Geometry check sheet. Reference: the model listing, model coordinates, mm. Face numbers are marked on the shaded views. A direction names the side the tool comes from. Give positions to 0.01 mm unless a question says otherwise; leave off trailing zeros. Write each loop counter-clockwise with the first axis right and the second up, starting at its lowest first coordinate (ties: lowest second). Pieces come first, ordered by that corner, then holes. Notation, with made-up numbers: M -28,9 L 10,9 A20 cw 10,35 Z; hole C 71.5,53 d8. An arc over 180 degrees is marked long. Write each question's results on one line, items separated by ' | '.
```python
from build123d import *

# Parameters (mm, degrees)
EXTRUDE1_DEPTH                   = 15.875
EXTRUDE2_DEPTH                   = 50
F_3_8_0_375_DIAMETER_HOLE1_D     = 9.525
F_3_8_0_375_DIAMETER_HOLE1_DEPTH = 32.4000114
F_3_8_0_375_DIAMETER_HOLE1_TIP   = 1.733408241
SKETCH6_R                        = 4.5
EXTRUDE3_DEPTH                   = 165.426993678


with BuildPart() as part:
    # Sketch1 → Extrude1 (new body)
    with BuildSketch(Plane(origin=(0, 0, 0), x_dir=(0, 0, -1), z_dir=(1, 0, 0))):
        with BuildLine():
            Line((0, 0), (-155.575, 0))
            Line((-155.575, 0), (-155.575, 14.6939))
            Line((-155.575, 14.6939), (-76.581, 14.6939))
            ThreePointArc((-76.581, 14.6939), (-69.845807909, 17.483707909), (-67.056, 24.2189))
            Line((-67.056, 24.2189), (-67.056, 25.4254))
            ThreePointArc((-67.056, 25.4254), (-69.845807909, 32.160592091), (-76.581, 34.9504))
            Line((-76.581, 34.9504), (-89.706369343, 34.9504))
            Line((-89.706369343, 34.9504), (-92.456, 36.5379))
            Line((-92.456, 36.5379), (-92.456, 49.2125))
            Line((-92.456, 49.2125), (-89.706369343, 50.8))
            Line((-89.706369343, 50.8), (0, 50.8))
            Line((0, 50.8), (0, 0))
        make_face()
    extrude(amount=EXTRUDE1_DEPTH)

    # Sketch2 → Extrude2 (cut)
    with BuildSketch(Plane.XY.offset(155.575)):
        Polygon((0, 10.9855), (4.462954262, 10.9855), (6.604, 14.6939), (9.271, 14.6939), (11.412045738, 10.9855), (15.875, 10.9855), (15.875, 23.6855), (0, 23.6855), align=None)
    extrude(amount=-EXTRUDE2_DEPTH, mode=Mode.SUBTRACT)

    # Sketch3 → Cut-Revolve1 (revolve, cut)
    with BuildSketch(Plane.XY.offset(105.575)):
        Polygon((0, 10.9855), (4.462954262, 10.9855), (6.604, 14.6939), (9.271, 14.6939), (11.412045738, 10.9855), (15.875, 10.9855), (15.875, 23.6855), (0, 23.6855), align=None)
    revolve(axis=Axis((15.875, 23.6855, 105.575), (-1, 0, 0)), mode=Mode.SUBTRACT)

    # 3/8 (0.375) Diameter Hole1
    with Locations(Plane(origin=(0, 50.8, 0), x_dir=(-1, 0, 0), z_dir=(0, 1, 0))):
        with Locations((-7.9375, 25.4), (-7.9375, 12.7)):
            Hole(F_3_8_0_375_DIAMETER_HOLE1_D / 2, depth=F_3_8_0_375_DIAMETER_HOLE1_DEPTH)
            with Locations((0, 0, -(F_3_8_0_375_DIAMETER_HOLE1_DEPTH + F_3_8_0_375_DIAMETER_HOLE1_TIP / 2))):  # 140° drill point
                Cone(0, F_3_8_0_375_DIAMETER_HOLE1_D / 2, F_3_8_0_375_DIAMETER_HOLE1_TIP, mode=Mode.SUBTRACT)

    # Sketch6 → Extrude3 (cut, through all)
    with BuildSketch(Plane(origin=(15.875, 0, 0), x_dir=(0, 0, -1), z_dir=(1, 0, 0))):
        with Locations((-54.230000076, 12.609999896)):
            Circle(SKETCH6_R)
        with Locations((-19.230000076, 12.609999896)):
            Circle(SKETCH6_R)
        with Locations((-59.980000078, 42.60999987)):
            Circle(SKETCH6_R)
        Polygon((-155.575, 8.3439), (-144.576477372, 14.6939), (-155.575, 14.6939), align=None)
    extrude(amount=-EXTRUDE3_DEPTH, mode=Mode.SUBTRACT)


solid = part.part
```
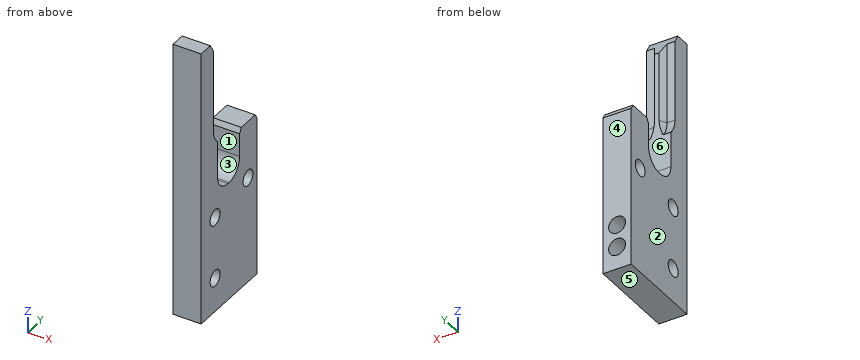
Q1. Access from +Z, -Z, +X, -X, +Y, -Y to the whole of each face (thin tool, end or side, straight path). Record for the marked faces 1 and 2.
Answer key:
face 1: +Z, +X, -X | face 2: +Z, -Z, -X, +Y, -Y
Q2. Material ranges on probe 1 along X at (y, z) = (43.5, 12.7) (3 decimals); probe 2 along Z at (x, y) = (12.25, 41); probe 3 along Z at (x, y) = (8.75, 42.61), recorded low to high. Write a range as [from, to].
Answer key:
probe 1: x = [0, 3.175], [12.7, 15.875] | probe 2: z = [0, 10.68], [14.72, 23.38], [27.42, 55.78], [64.18, 92.46] | probe 3: z = [0, 8.01], [17.39, 20.71], [30.09, 55.48], [64.48, 92.46]
Q3. Section check C-C (z = 133). Enter the section's corners in (x, y) (1 decimal).
Answer key:
outline: M 0,0 L 15.9,0 L 15.9,11 L 11.4,11 L 9.3,14.7 L 6.6,14.7 L 4.5,11 L 0,11 Z
Q4. Section check A-A (y = 42.61). Enter the section's corners in (x, z) (1 decimal), then the cut area to 3 significant figures.
Answer key:
outline: M 0,0 L 15.9,0 L 15.9,55.5 L 0,55.5 Z; M 0,64.5 L 15.9,64.5 L 15.9,92.5 L 0,92.5 Z; hole C 7.9,12.7 d9.5; hole C 7.9,25.4 d9.5 | area: 1,180 mm2
Q5. Depth check by flat-ended pin: P1, Ø1, axis at y = 44, z = 71, coming from the -X side; P2, Ø5, axis at x = 4, z = 123, coming from the +Y side; P3, Ø1, axis at x = 6.5, y = 15, coming from the +Z side; P4, Ø6, axis at x = 11, y = 34, coming from the +Z side. Enter the tip coordinate at first touch or a pass-through.
Answer key:
P1: stops at x = 0 | P2: stops at y = 14.51 | P3: stops at z = 144.91 | P4: stops at z = 92.46
Q6. Section check D-D (y = 30). Enter the section's corners in (x, z) (1 decimal), then the cut area to 3 significant figures.
Answer key:
outline: M 0,0 L 15.9,0 L 15.9,68.2 L 0,68.2 Z; hole C 7.9,12.7 d9.5; hole C 7.9,25.4 d9.5 | area: 941 mm2
Q7. Release check for a two-part mould opening along Y. For the marked faces 3, 4, 5 and 6 record: released by +Y, released by -Y, zero draft, split by the parting line, or undercut.
Answer key:
face 3: undercut | face 4: released by +Y | face 5: zero draft | face 6: undercut
Q8. Section check B-B (z = 19.23). Enter the section's corners in (x, y) (3 decimals).
Answer key:
outline: M 0,0 L 15.875,0 L 15.875,8.11 L 0,8.11 Z; M 0,17.11 L 15.875,17.11 L 15.875,50.8 L 0,50.8 Z
